Geometry check sheet. Reference: the model listing, model coordinates, mm. Face numbers are marked on the shaded views. A direction names the side the tool comes from. Round coordinates to 2 decimals unless told otherwise and drop trailing zeros. Order: outer loops, then holes, each group sorted by start corner. A loop starts at its lowest first (then second) coordinate and runs counter-clockwise, first axis right, second up.
(1) Release check for a two-part mould opening along X. For the marked faces 4, 5 and 6 record: +X half, -X half, draft (parallel to the pull), parting line (faces both ways), or undercut.
(2) Go/stop test with flat-tipped pins: pin 1 (5.5 mm diameter, centred on y = 47, z = -20.5, fed in from -X); pin 2 (4.5 mm diameter, centred on x = 47.5, z = -15, fed in from -Y); pin 3 (4 mm diameter, centred on x = 45, z = -26.5, fed in from +Y); pin 4 (3 mm diameter, centred on x = 45.5, y = 45.5, fed in from +Z). Record where each tip stops, or that it passes through.
(3) Sectioned sample at C-C (y = 52.5). Give the number of separate pieces and of enclosed holes in the cut face, plus the area to 3 significant figures.
(4) Sectioned sample at B-B (x = 45.5). Record the boundary of the cut face in (y, z), plus the area to 3 significant figures.
(5) Material ranges on line 1 along X through (y, z) = (52.6, -13); line 2 along Y through (x, z) = (45, -28.25); line 3 along X through (y, z) = (41.15, -26), recorded low to high.
(6) Sectioned sample at A-A (z = -13). Record the boundary of the cut face in (x, y).
(7) Set-up check for the marked faces 1, 2 and 3: record each of +Z, -Z, +X, -X, +Y, -Y from which the full face is reachable in a straight line by a thin tool's end or side.
(8) Sectioned sample at D-D (x = 49.5). Record the boundary of the cut face in (y, z).
from build123d import *

# Parameters (mm, degrees)
CYLINDER730_R          = 3.1
CYLINDER730_DEPTH      = 2
CYLINDER730_ROLL_ANGLE = 90
CYLINDER726_R          = 2.1
CYLINDER726_DEPTH      = 15
CYLINDER726_ROLL_ANGLE = 90
CYLINDER728_R          = 1.6
CYLINDER728_DEPTH      = 15
CYLINDER728_ROLL_ANGLE = 90
CYLINDER727_R          = 1.6
CYLINDER727_DEPTH      = 15
CYLINDER727_ROLL_ANGLE = 90
CYLINDER729_R          = 3.1
CYLINDER729_DEPTH      = 2
CYLINDER729_ROLL_ANGLE = 90
BOX483_W               = 12
BOX483_H               = 7.5
BOX483_DEPTH           = 8
BOX482_W               = 12
BOX482_H               = 13.75
BOX482_DEPTH           = 12
BOX484_W               = 16
BOX484_H               = 3.75
BOX484_DEPTH           = 10
FILLET334_R            = 3
FILLET335_R            = 4
CHAMFER081_SIZE        = 1.99


with BuildPart() as cylinder837:
    # Cylinder730 → Cylinder730 (new body)
    with BuildSketch(Plane.XY):
        Circle(CYLINDER730_R)
    extrude(amount=CYLINDER730_DEPTH)


with BuildPart() as cylinder837_1:
    # Cylinder730 roll: moved
    add(cylinder837.part.rotate(Axis((0, 0, 0), (1, 0, 0)), CYLINDER730_ROLL_ANGLE))


with BuildPart() as cylinder837_2:
    # Cylinder730 placement: moved
    add(cylinder837_1.part.moved(Location((399.5, 49.75, -15))))


with BuildPart() as cylinder833:
    # Cylinder726 → Cylinder726 (new body)
    with BuildSketch(Plane.XY):
        Circle(CYLINDER726_R)
    extrude(amount=CYLINDER726_DEPTH)


with BuildPart() as cylinder833_1:
    # Cylinder726 roll: moved
    add(cylinder833.part.rotate(Axis((0, 0, 0), (1, 0, 0)), CYLINDER726_ROLL_ANGLE))


with BuildPart() as cylinder833_2:
    # Cylinder726 placement: moved
    add(cylinder833_1.part.moved(Location((395.5, 54, -28))))


with BuildPart() as cylinder835:
    # Cylinder728 → Cylinder728 (new body)
    with BuildSketch(Plane.XY):
        Circle(CYLINDER728_R)
    extrude(amount=CYLINDER728_DEPTH)


with BuildPart() as cylinder835_1:
    # Cylinder728 roll: moved
    add(cylinder835.part.rotate(Axis((0, 0, 0), (1, 0, 0)), CYLINDER728_ROLL_ANGLE))


with BuildPart() as cylinder835_2:
    # Cylinder728 placement: moved
    add(cylinder835_1.part.moved(Location((399.5, 54, -15))))


with BuildPart() as cylinder834:
    # Cylinder727 → Cylinder727 (new body)
    with BuildSketch(Plane.XY):
        Circle(CYLINDER727_R)
    extrude(amount=CYLINDER727_DEPTH)


with BuildPart() as cylinder834_1:
    # Cylinder727 roll: moved
    add(cylinder834.part.rotate(Axis((0, 0, 0), (1, 0, 0)), CYLINDER727_ROLL_ANGLE))


with BuildPart() as cylinder834_2:
    # Cylinder727 placement: moved
    add(cylinder834_1.part.moved(Location((391.5, 54, -15))))


with BuildPart() as fusion476:
    # Cylinder729 → Cylinder729 (new body)
    with BuildSketch(Plane.XY):
        Circle(CYLINDER729_R)
    extrude(amount=CYLINDER729_DEPTH)


with BuildPart() as fusion476_1:
    # Cylinder729 roll: moved
    add(fusion476.part.rotate(Axis((0, 0, 0), (1, 0, 0)), CYLINDER729_ROLL_ANGLE))


with BuildPart() as fusion476_2:
    # Cylinder729 placement: moved
    add(fusion476_1.part.moved(Location((391.5, 49.75, -15))))

    # Fusion476: union Cylinder837, Cylinder833, Cylinder835, Cylinder834
    add(cylinder837_2.part)
    add(cylinder833_2.part)
    add(cylinder835_2.part)
    add(cylinder834_2.part)


with BuildPart() as cube685:
    # Box483 → Box483 (new body)
    with BuildSketch(Plane(origin=(389.5, 41.75, -32), x_dir=(1, 0, 0), z_dir=(0, 0, 1))):
        with Locations((6, 3.75)):
            Rectangle(BOX483_W, BOX483_H)
    extrude(amount=BOX483_DEPTH)


with BuildPart() as cut873:
    # Box482 → Box482 (new body)
    with BuildSketch(Plane(origin=(389.5, 39.75, -32), x_dir=(1, 0, 0), z_dir=(0, 0, 1))):
        with Locations((6, 6.875)):
            Rectangle(BOX482_W, BOX482_H)
    extrude(amount=BOX482_DEPTH)

    # Cut594: cut Cube685
    add(cube685.part, mode=Mode.SUBTRACT)


with BuildPart() as obj1:
    # Box484 → Box484 (new body)
    with BuildSketch(Plane(origin=(387.5, 49.75, -20), x_dir=(1, 0, 0), z_dir=(0, 0, 1))):
        with Locations((8, 1.875)):
            Rectangle(BOX484_W, BOX484_H)
    extrude(amount=BOX484_DEPTH)

    # Fusion475: union Cut873
    add(cut873.part)

    # Fillet334
    fillet334_edges = [obj1.edges().sort_by_distance(p)[0] for p in [
        (395.5, 49.75, -20),
        (395.5, 49.75, -10),
        (395.5, 39.75, -20),
    ]]
    fillet(fillet334_edges, radius=FILLET334_R)

    # Fillet335
    fillet335_edges = [obj1.edges().sort_by_distance(p)[0] for p in [
        (389.5, 40.75, -32),
        (389.5, 51.375, -32),
        (401.5, 40.75, -32),
        (401.5, 51.375, -32),
    ]]
    fillet(fillet335_edges, radius=FILLET335_R)

    # Chamfer081
    chamfer081_edges = [obj1.edges().sort_by_distance(p)[0] for p in [
        (401.5, 51.625, -20),
        (389.5, 51.625, -20),
    ]]
    chamfer(chamfer081_edges, length=CHAMFER081_SIZE)

    # Cut593: cut Fusion476
    add(fusion476_2.part, mode=Mode.SUBTRACT)


with BuildPart() as obj1_1:
    # Cut593 placement: moved
    add(obj1.part.moved(Location((-350, 0, 2))))


solid = obj1_1.part
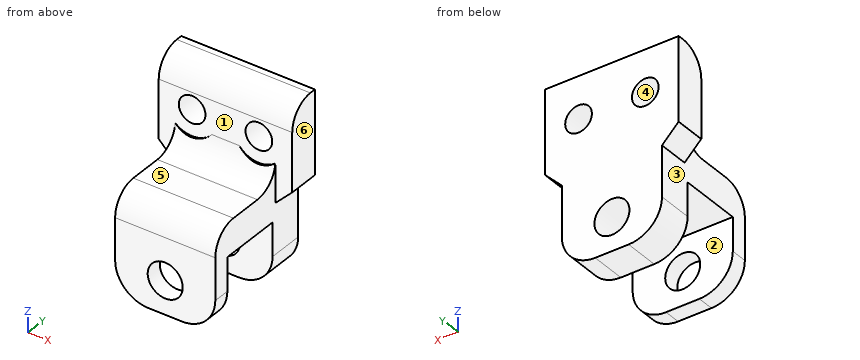
Answer below:
1. face 4: undercut
1. face 5: draft
1. face 6: +X half
2. pin 1: stops at x = 39.5
2. pin 2: stops at y = 48.73
2. pin 3: stops at y = 53.5
2. pin 4: stops at z = -17.99
3. separate pieces: 1
3. enclosed holes: 3
3. area: 271 mm2
4. outline: (39.75, -30) - (41.75, -30) - (41.75, -28.1) - (39.75, -28.1) - close; (39.75, -23.9) - (41.75, -23.9) - (41.75, -22) - (49.25, -22) - (49.25, -23.9) - (53.5, -23.9) - (53.5, -8) - (52.75, -8) arc R3 ccw to (49.75, -11) - (49.75, -15) arc R3 cw to (46.75, -18) - (42.75, -18) arc R3 ccw to (39.75, -21) - close; (49.25, -30) - (53.5, -30) - (53.5, -28.1) - (49.25, -28.1) - close
4. area: 114 mm2
5. line 1: x = 37.5 to 39.9, 43.1 to 47.9, 51.1 to 53.5
5. line 2: y = 39.75 to 41.75, 49.25 to 53.5
5. line 3: x = 39.5 to 43.4, 47.6 to 51.5
6. outline: (37.5, 49.75) - (39.9, 49.75) - (39.9, 53.5) - (37.5, 53.5) - close; (43.1, 49.75) - (47.9, 49.75) - (47.9, 53.5) - (43.1, 53.5) - close; (51.1, 49.75) - (53.5, 49.75) - (53.5, 53.5) - (51.1, 53.5) - close
7. face 1: +Z, -Y
7. face 2: -Z, +X, -X
7. face 3: -Z, -X, -Y
8. outline: (39.75, -29.46) - (41.75, -29.46) - (41.75, -22) - (49.25, -22) - (49.25, -29.46) - (53.5, -29.46) - (53.5, -14.6) - (49.75, -14.6) - (49.75, -16.1) - (49.54, -16.1) arc R3 cw to (46.75, -18) - (42.75, -18) arc R3 ccw to (39.75, -21) - close; (49.75, -11.4) - (53.5, -11.4) - (53.5, -8) - (52.75, -8) arc R3 ccw to (49.75, -11) - close
